Check sheet for the drawn part. Datum: minimum x, y, z corner. Units: mm. Coordinates: 2 decimals unless noted, no trailing zeros. Write each loop counter-clockwise with the first axis right and the second up, starting at its lowest first coordinate (ties: lowest second). Pieces come first, ordered by that corner, then holes. Notation, with made-up numbers: (10, 70.25) - (45, 70.25) arc R23 ccw to (45, 103.25) - close; hole circle Ø1 at (28.25, 54.25). An arc over 180 degrees is marked (long way). Answer as CSV lines item,"result". Start each with the question number.
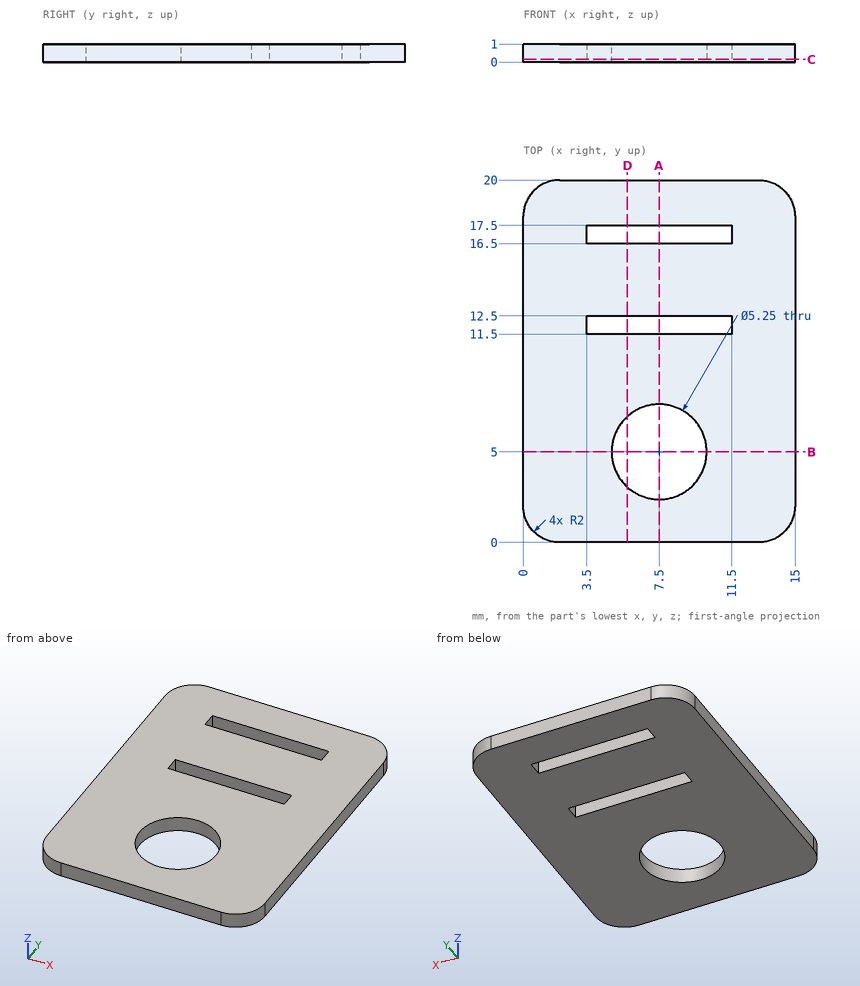
(1) Cross-section at A-A on x = 7.5. Record the boundary of the cut face in (y, z) (3 decimals), plus the area to 4 significant figures.
(2) Material ranges on probe 1 along Y at (x, z) = (7.5, 0.4) (3 decimals); probe 2 along X at (y, z) = (12.25, 0.9); probe 3 along Y at (x, z) = (6.5, 0.85), recorded low to high. Write a range as from..to.
(3) Cross-section at D-D on x = 5.75. Record the boundary of the cut face in (y, z), plus the area to 3 significant figures.
(4) Cross-section at C-C on z = 0.15. Record the boundary of the cut face in (x, y) (3 decimals).
(5) Cross-section at B-B on y = 5. Record the boundary of the cut face in (x, z) (3 decimals), plus the area to 3 significant figures.
Checked values:
1,outline,"(0, 0) - (2.375, 0) - (2.375, 1) - (0, 1) - close; (7.625, 0) - (11.5, 0) - (11.5, 1) - (7.625, 1) - close; (12.5, 0) - (16.5, 0) - (16.5, 1) - (12.5, 1) - close; (17.5, 0) - (20, 0) - (20, 1) - (17.5, 1) - close"
1,area,"12.75 mm^2"
2,probe 1,"0..2.375, 7.625..11.5, 12.5..16.5, 17.5..20"
2,probe 2,"0..3.5, 11.5..15"
2,probe 3,"0..2.57, 7.43..11.5, 12.5..16.5, 17.5..20"
3,outline,"(0, 0) - (3.04, 0) - (3.04, 1) - (0, 1) - close; (6.96, 0) - (11.5, 0) - (11.5, 1) - (6.96, 1) - close; (12.5, 0) - (16.5, 0) - (16.5, 1) - (12.5, 1) - close; (17.5, 0) - (20, 0) - (20, 1) - (17.5, 1) - close"
3,area,"14.1 mm^2"
4,outline,"(0, 2) arc R2 ccw to (2, 0) - (13, 0) arc R2 ccw to (15, 2) - (15, 18) arc R2 ccw to (13, 20) - (2, 20) arc R2 ccw to (0, 18) - close; hole (3.5, 11.5) - (11.5, 11.5) - (11.5, 12.5) - (3.5, 12.5) - close; hole (3.5, 16.5) - (11.5, 16.5) - (11.5, 17.5) - (3.5, 17.5) - close; hole circle Ø5.25 at (7.5, 5)"
5,outline,"(0, 0) - (4.875, 0) - (4.875, 1) - (0, 1) - close; (10.125, 0) - (15, 0) - (15, 1) - (10.125, 1) - close"
5,area,"9.75 mm^2"
